from build123d import *

# Parameters (mm, degrees)
BOSS_EXTRUDE1_DEPTH = 20
SKETCH2_R           = 2.5
CUT_EXTRUDE1_DEPTH  = 23


with BuildPart() as part:
    # Sketch1 → Boss-Extrude1 (new body)
    with BuildSketch(Plane.XY):
        Polygon((0, 0), (60, 0), (60, 20), (50.15, 20), (50.15, 22), (9.85, 22), (9.85, 20), (0, 20), align=None)
    extrude(amount=BOSS_EXTRUDE1_DEPTH)

    # Sketch2 → Cut-Extrude1 (cut, through all)
    with BuildSketch(Plane.XZ):
        with Locations((55, 5)):
            Circle(SKETCH2_R)
        with Locations((5, 5)):
            Circle(SKETCH2_R)
    extrude(amount=-CUT_EXTRUDE1_DEPTH, mode=Mode.SUBTRACT)


solid = part.part
Geometry: final body of the model. Coordinates: model frame, mm. A direction names the side the tool comes from. Coordinates: 2 decimals unless noted, no trailing zeros. Order: outer loops, then holes, each group sorted by start corner. A loop starts at its lowest first (then second) coordinate and runs counter-clockwise, first axis right, second up. Notation, with made-up numbers: (72.5, 64.25) - (92.5, 64.25) arc R26 cw to (92.5, 97.25) - close; hole circle Ø4 at (50.25, 13.5). An arc over 180 degrees is marked (long way). Use one line per item in the form item = value.
1) Section A-A (x = 55). Return loops of the section in (y, z), then the cut area to 3 significant figures.
Solutions:
outline = (0, 0) - (20, 0) - (20, 2.5) - (0, 2.5) - close; (0, 7.5) - (20, 7.5) - (20, 20) - (0, 20) - close
area = 300 mm^2
2) Mould query, pull axis X, two halves, no side actions, for faces 3 (the face through (9.85, 21, 10)), 4 (the face through (57.31, 9.86, 4.04)), 5 (the face through (60, 10, 10)), 6 (the face through (5, 20, 10)). Classes: +X half, -X half, draft (parallel to the pull), parting line (faces both ways), or undercut.
Solutions:
face_3 = -X half
face_4 = undercut
face_5 = +X half
face_6 = draft
3) Ray query, L1, parallel to Z at x = 55, y = 9.75; L2, parallel to X at y = 21.25, z = 18.5; L3, parallel to Y at x = 7, z = 13. Return the intervals inside material, ascending.
Solutions:
L1 = 0 to 2.5, 7.5 to 20
L2 = 9.85 to 50.15
L3 = 0 to 20
4) Pin query (flat end, axial travel): pin 1 (2 mm diameter, centred on x = 30.5, y = 16, fed in from -Z); pin 2 (8 mm diameter, centred on x = 5, z = 5, fed in from +Y); pin 3 (0.6 mm diameter, centred on y = 21, z = 11.5, fed in from +X). Return the tip coordinate at first contact, or that it passes through.
Solutions:
pin_1 = 0
pin_2 = 20
pin_3 = 50.15
5) Section D-D (y = 6.25). Return loops of the section in (x, z).
Solutions:
outline = (0, 0) - (60, 0) - (60, 20) - (0, 20) - close; hole circle Ø5 at (5, 5); hole circle Ø5 at (55, 5)
6) Section C-C (z = 15.75). Return loops of the section in (x, y).
Solutions:
outline = (0, 0) - (60, 0) - (60, 20) - (50.15, 20) - (50.15, 22) - (9.85, 22) - (9.85, 20) - (0, 20) - close
7) Section B-B (z = 5). Return loops of the section in (x, y), then the cut area to 3 significant figures.
Solutions:
outline = (0, 0) - (2.5, 0) - (2.5, 20) - (0, 20) - close; (7.5, 0) - (52.5, 0) - (52.5, 20) - (50.15, 20) - (50.15, 22) - (9.85, 22) - (9.85, 20) - (7.5, 20) - close; (57.5, 0) - (60, 0) - (60, 20) - (57.5, 20) - close
area = 1,080 mm^2
8) Set-up query: faces 1 (the face through (55, 20, 10)), 2 (the face through (7.385, 9.86, 5.751)). Return all of +Z, -Z, +X, -X, +Y, -Y with unobstructed straight access to the full face (end or side cutting, diameter ignored); none if empty.
Solutions:
face_1 = +Z, -Z, +X, +Y
face_2 = +Y, -Y
